Read the model definition and answer for the solid it produces. Units are mm, in the model's axes. Round coordinates to 2 decimals unless told otherwise and drop trailing zeros. Loops run counter-clockwise (first coordinate to the right, second up) from the corner with the lowest first, then second, coordinate; pieces in that order, holes last. Notation, with made-up numbers: (-39, 20) - (-35, 20) arc R28 cw to (-35, 54) - close; hole circle Ø2 at (35, -19.75). An arc over 180 degrees is marked (long way). Answer as CSV lines item,"result".
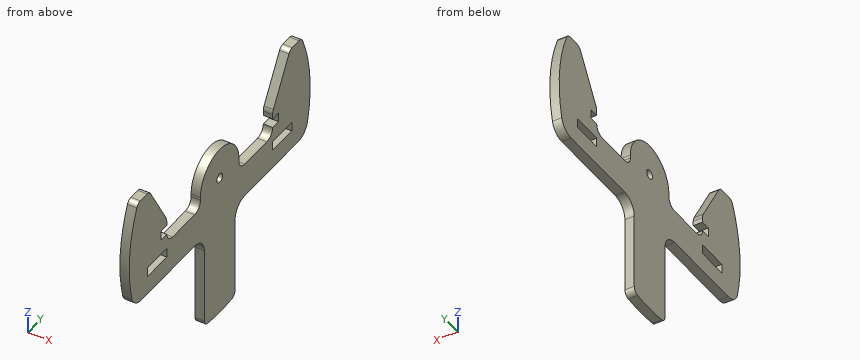
Autodesk Inventor part; units mm, degrees
ref_plane "YZ Plane" through (0, 0, 0) normal (1, 0, 0) x (0, 1, 0)
ref_plane "XZ Plane" through (0, 0, 0) normal (0, 1, 0) x (-1, 0, 0)
ref_plane "XY Plane" through (0, 0, 0) normal (0, 0, 1) x (1, 0, 0)
sketch "Sketch1" plane through (0, 0, 0) normal (1, 0, 0) x (0, 1, 0)
  line L0 (-46.6154, -6) -> (46.6154, -6) construction
  line L1 (-37.5, -6) -> (-27.5, -6)
  line L2 (-27.5, -6) -> (-27.5, -9)
  line L3 (-27.5, -9) -> (-37.5, -9)
  line L4 (-37.5, -9) -> (-37.5, -6)
  line L5 (27.5, -6) -> (37.5, -6)
  line L6 (37.5, -6) -> (37.5, -9)
  line L7 (37.5, -9) -> (27.5, -9)
  line L8 (27.5, -9) -> (27.5, -6)
  arc A0 (10, 0) -> (-10, 0) centre (0, 0) ccw
  circle A1 centre (0, 0) radius 1.5
  line L9 (-35.955, 19) -> (-27.9019, 5.0517)
  line L10 (27.9019, 5.0517) -> (35.955, 19)
  line L11 (-8, -44.5982) -> (-8, -20)
  line L12 (8, -44.5982) -> (8, -20)
  arc A2 (-6.2667, -46.5803) -> (6.2667, -46.5803) centre (0, 0) ccw
  line L13 (-25, -39.7995) -> (25, -39.7995) construction
  line L14 (40.7922, -15) -> (13, -15)
  line L15 (-40.8058, -15) -> (-13, -15)
  arc A3 (45.6484, -11.1905) -> (43.0762, 18.8) centre (0, 0) ccw
  line L16 (-46.7846, 0) -> (47, 0) construction
  arc A4 (-45.5561, -11.5602) -> (-40.8058, -15) centre (-40.8058, -10) ccw
  arc A5 (40.7922, -15) -> (45.6484, -11.1905) centre (40.7922, -10) ccw
  arc A6 (-43.0762, 18.8) -> (-45.5561, -11.5602) centre (0, 0) ccw
  line L17 (-41.2432, 20) -> (-37.687, 20)
  line L18 (37.687, 20) -> (41.2432, 20)
  arc A7 (-41.2432, 20) -> (-43.0762, 18.8) centre (-41.2432, 18) ccw
  arc A8 (-35.955, 19) -> (-37.687, 20) centre (-37.687, 18) ccw
  arc A9 (43.0762, 18.8) -> (41.2432, 20) centre (41.2432, 18) ccw
  arc A10 (37.687, 20) -> (35.955, 19) centre (37.687, 18) ccw
  line L19 (-27.5, -1) -> (-30.5, -1)
  line L20 (-30.5, -1) -> (-30.5, 2)
  line L21 (-30.5, 2) -> (-27.5, 2)
  line L22 (27.5, -1) -> (30.5, -1)
  line L23 (30.5, -1) -> (30.5, 2)
  line L24 (30.5, 2) -> (27.5, 2)
  arc A11 (-8, -44.5982) -> (-6.2667, -46.5803) centre (-6, -44.5982) ccw
  arc A12 (6.2667, -46.5803) -> (8, -44.5982) centre (6, -44.5982) ccw
  line L25 (-27.5, 2) -> (-27.5, 3.5517)
  line L26 (27.5, 2) -> (27.5, 3.5517)
  line L27 (-27.5, -1) -> (-27.5, -1)
  line L28 (27.5, -1) -> (27.5, -1)
  line L29 (-10, 0) -> (-10, -1)
  line L30 (10, 0) -> (10, -1)
  line L31 (-24.5, -4) -> (-13, -4)
  line L32 (13, -4) -> (24.5, -4)
  arc A13 (-27.5, -1) -> (-24.5, -4) centre (-24.5, -1) ccw
  arc A14 (-27.5, 3.5517) -> (-27.9019, 5.0517) centre (-30.5, 3.5517) ccw
  arc A15 (-13, -4) -> (-10, -1) centre (-13, -1) ccw
  arc A16 (10, -1) -> (13, -4) centre (13, -1) ccw
  arc A17 (24.5, -4) -> (27.5, -1) centre (24.5, -1) ccw
  arc A18 (27.9019, 5.0517) -> (27.5, 3.5517) centre (30.5, 3.5517) ccw
  arc A19 (-8, -20) -> (-13, -15) centre (-13, -20) ccw
  arc A20 (13, -15) -> (8, -20) centre (13, -20) ccw
  point P0 (-42.5323, 20)
  point P1 (42.5323, 20)
  point P2 (-36.5323, 20)
  point P3 (36.5323, 20)
  point P4 (-26.14, 2)
  point P5 (26.14, 2)
  point P6 (-8, -10)
  point P7 (8, -10)
  point P8 (-45.4579, -15)
  point P9 (44.5421, -15)
  point P10 (-25.4579, -10)
  point P11 (8, -15)
  point P12 (-8, -15)
  point P13 (-8, -46.3141)
  point P14 (8, -46.3141)
  dimension "d3" = 10
  dimension "d4" = 3
  dimension "d5" = 10
  dimension "d6" = 3
  dimension "d105" = 50
  dimension "d116" = 6
  dimension "d122" = 8
  dimension "d123" = 8
  dimension "d131" = 47
  dimension "d137" = 5
  dimension "d141" = 6
  dimension "d142" = 120
  dimension "d143" = 6
  dimension "d144" = 120
  dimension "d145" = 2
  dimension "d146" = 3
  dimension "d147" = 3
  dimension "d148" = 5
  dimension "d149" = 3
  dimension "d150" = 3
  dimension "d151" = 5
  dimension "d154" = 47
  dimension "d155" = 10
  dimension "d156" = 2
  dimension "d159" = 20
  dimension "d160" = 20
  dimension "d162" = 3
  dimension "d163" = 15
  dimension "d164" = 15
  dimension "d167" = 30.5
  dimension "d168" = 30.5
  dimension "d169" = 3
  dimension "d170" = 3
  dimension "d171" = 27.5
  dimension "d172" = 27.5
  dimension "d173" = 5
  dimension "d174" = 11
  dimension "d175" = 11
extrude "Extrusion5" add sketch "Sketch1" along normal blind 3
properties part number "Endplate 072313"
1) A cutting plane is placed at A-A, the plane y = 0. Determine the outline of the cut face in (x, z).
Entries:
outline,"(0, -47) - (3, -47) - (3, -1.5) - (0, -1.5) - close; (0, 1.5) - (3, 1.5) - (3, 10) - (0, 10) - close"
2) A cutting plane is placed at D-D, the plane y = -33.5. Determine the outline of the cut face in (x, z), plus the area to 3 significant figures.
Entries:
outline,"(0, -15) - (3, -15) - (3, -9) - (0, -9) - close; (0, -6) - (3, -6) - (3, 14.75) - (0, 14.75) - close"
area,"80.2 mm^2"
3) Each of these flat-tipped pins is pushed along its axis until it touches: P1, Ø1.5, axis at x = 1.5, y = 35, coming from the +Z side; P2, Ø1, axis at x = 2.5, y = -22, coming from the -Z side; P3, Ø0.8, axis at x = 2, z = 2.5, coming from the -Y side. Where does it stop, or does it pass through?
Entries:
P1,"stops at z = 18.64"
P2,"stops at z = -15"
P3,"stops at y = -46.95"
4) Find the intervals of material crossed by line 1 (Z direction, x = 1.1, y = 0); line 2 (Z direction, x = 1.55, y = 30); line 3 (Y direction, x = 0.4, z = -8), in increasing order.
Entries:
line 1,"z = -47 to -1.5, 1.5 to 10"
line 2,"z = -15 to -9, -6 to -1, 2 to 8.69"
line 3,"y = -46.31 to -37.5, -27.5 to 27.5, 37.5 to 46.31"
5) A cutting plane is placed at B-B, the plane z = -7. Determine the outline of the cut face in (x, y), plus the area to 3 significant figures.
Entries:
outline,"(0, -46.48) - (3, -46.48) - (3, -37.5) - (0, -37.5) - close; (0, -27.5) - (3, -27.5) - (3, 27.5) - (0, 27.5) - close; (0, 37.5) - (3, 37.5) - (3, 46.48) - (0, 46.48) - close"
area,"219 mm^2"
6) A cutting plane is placed at C-C, the plane x = 1.75. Count the separate pieces of the cut face and the enclosed holes in it, plus the area to 3 significant figures.
Entries:
separate pieces,"1"
enclosed holes,"3"
area,"2,420 mm^2"
